CAD build for the part. Positions are in the model's coordinates, mm. Face numbers are marked on the shaded views. A direction names the side the tool comes from. Round coordinates to 2 decimals unless told otherwise and drop trailing zeros. Write each loop counter-clockwise with the first axis right and the second up, starting at its lowest first coordinate (ties: lowest second). Pieces come first, ordered by that corner, then holes. Notation, with made-up numbers: (41, 38.5) - (69, 38.5) arc R12 ccw to (69, 55.5) - close; hole circle Ø4 at (-40, 25). An arc over 180 degrees is marked (long way). Answer in a Markdown table with one row per item.
```python
from build123d import *

# Parameters (mm, degrees)
MOTOR_MOUNT_SOLID_DEPTH              = 7.5
ENCODER_DISTANCE_SKETCH_W            = 50
ENCODER_DISTANCE_SKETCH_H            = 55
ENCODER_DISTANCE_SOLID_DEPTH         = 5
ENCODER_MOUNT_SKETCH_R               = 1.9
ENCODER_MOUNT_SKETCH_W               = 7
ENCODER_MOUNT_SKETCH_H               = 9
ENCODER_MOUNT_SOLID_DEPTH            = 5
MOTOR_CLAMP_MOUNTING_HOLES_SKETCH_R  = 1.9
MOTOR_CLAMP_MOUNTING_HOLES_CUT_DEPTH = 16
GUSSET_PLATE_SKETCH_W                = 50
GUSSET_PLATE_SKETCH_H                = 5
GUSSET_PLATE_SOLID_DEPTH             = 16.5
GUSSET_SOLID_DEPTH                   = 1.5
MOUNTING_PLATE_SKETCH_W              = 50
MOUNTING_PLATE_SKETCH_H              = 92
MOUNTING_PLATE_SKETCH_R              = 2.65
MOUNTING_PLATE_SOLID_DEPTH           = 5
MOUNTING_HOLES_CUT_DEPTH             = 100.036609393
MOUNTING_HOLES_CUT_DEPTH_BACK        = 100.036609393
MOUNTING_HOLE_SKETCH_R               = 2.65
MOUNTING_PLATE_TRIM_SKETCH_W         = 50
MOUNTING_PLATE_TRIM_SKETCH_H         = 15.5
MOUNTING_PLATE_TRIM_SKETCH_H_2       = 40
MOUNTING_PLATE_TRIM_SKETCH_W_2       = 23.5
MOUNTING_PLATE_TRIM_SKETCH_H_3       = 16.5
MOUNTING_PLATE_TRIM_CUT_DEPTH        = 2


with BuildPart() as part:
    # Mouting Mount Sketch → Motor Mount Solid (new, symmetric)
    with BuildSketch(Plane.XY):
        with BuildLine():
            Line((-25, -55), (25, -55))
            Line((25, -55), (25, 0))
            Line((25, 0), (10, 0))
            ThreePointArc((10, 0), (0, -10), (-10, 0))
            Line((-10, 0), (-25, 0))
            Line((-25, 0), (-25, -55))
        make_face()
    extrude(amount=MOTOR_MOUNT_SOLID_DEPTH, both=True)

    # Encoder Distance Sketch → Encoder Distance Solid (add)
    with BuildSketch(Plane.XZ.offset(55)):
        with Locations((0, 20)):
            Rectangle(ENCODER_DISTANCE_SKETCH_W, ENCODER_DISTANCE_SKETCH_H)
    extrude(amount=ENCODER_DISTANCE_SOLID_DEPTH)

    # Encoder Mount Sketch → Encoder Mount Solid (add)
    with BuildSketch(Plane.XY.offset(47.5)):
        Polygon((-25, -60), (-25, -55), (-11.5, 11.5), (11.5, 11.5), (25, -55), (25, -60), align=None)
        with Locations((-8, 8)):
            Circle(ENCODER_MOUNT_SKETCH_R, mode=Mode.SUBTRACT)
        with Locations((8, 8)):
            Circle(ENCODER_MOUNT_SKETCH_R, mode=Mode.SUBTRACT)
        with Locations((-8, -8)):
            Circle(ENCODER_MOUNT_SKETCH_R, mode=Mode.SUBTRACT)
        with Locations((8, -8)):
            Circle(ENCODER_MOUNT_SKETCH_R, mode=Mode.SUBTRACT)
        with Locations((-8, 0)):
            Rectangle(ENCODER_MOUNT_SKETCH_W, ENCODER_MOUNT_SKETCH_H, mode=Mode.SUBTRACT)
        with Locations((8, 0)):
            Rectangle(ENCODER_MOUNT_SKETCH_W, ENCODER_MOUNT_SKETCH_H, mode=Mode.SUBTRACT)
    extrude(amount=ENCODER_MOUNT_SOLID_DEPTH)

    # Motor Clamp Mounting Holes Sketch → Motor Clamp Mounting Holes Cut (cut)
    with BuildSketch(Plane(origin=(0, 0, 0), x_dir=(1, 0, 0), z_dir=(0, 1, 0))):
        with Locations(Location((-15, 0, 0), (0, 0, 180))):
            Circle(MOTOR_CLAMP_MOUNTING_HOLES_SKETCH_R)
        with Locations(Location((15, 0, 0), (0, 0, 180))):
            Circle(MOTOR_CLAMP_MOUNTING_HOLES_SKETCH_R)
    extrude(amount=-MOTOR_CLAMP_MOUNTING_HOLES_CUT_DEPTH, mode=Mode.SUBTRACT)

    # Gusset Plate Sketch → Gusset Plate Solid (add)
    with BuildSketch(Plane.XY.offset(52.5)):
        with Locations((0, -57.5)):
            Rectangle(GUSSET_PLATE_SKETCH_W, GUSSET_PLATE_SKETCH_H)
    extrude(amount=GUSSET_PLATE_SOLID_DEPTH)

    # Gusset Sketch → Gusset Solid (add, symmetric)
    with BuildSketch(Plane(origin=(0, 0, 0), x_dir=(0, 0, -1), z_dir=(1, 0, 0))):
        Polygon((-52.5, 11.5), (-69, -55), (-52.5, -55), align=None)
    extrude(amount=GUSSET_SOLID_DEPTH, both=True)

    # Mounting Plate Sketch → Mounting Plate Solid (add)
    with BuildSketch(Plane(origin=(0, -55, 0), x_dir=(1, 0, 0), z_dir=(0, 1, 0))):
        with Locations((0, -23)):
            Rectangle(MOUNTING_PLATE_SKETCH_W, MOUNTING_PLATE_SKETCH_H)
        with Locations((-19, -63)):
            Circle(MOUNTING_PLATE_SKETCH_R, mode=Mode.SUBTRACT)
        with Locations((19, -63)):
            Circle(MOUNTING_PLATE_SKETCH_R, mode=Mode.SUBTRACT)
        with Locations(Location((-19, 17, 0), (0, 0, 270))):
            Circle(MOUNTING_PLATE_SKETCH_R, mode=Mode.SUBTRACT)
        with Locations(Location((19, 17, 0), (0, 0, 270))):
            Circle(MOUNTING_PLATE_SKETCH_R, mode=Mode.SUBTRACT)
    extrude(amount=-MOUNTING_PLATE_SOLID_DEPTH)

    # Mounting Hole Sketch → Mounting Holes Cut (cut, two sides: drawn at the far end of the back side and taken through both)
    with BuildSketch(Plane(origin=(0, -55, 0), x_dir=(1, 0, 0), z_dir=(0, 1, 0)).offset(-MOUNTING_HOLES_CUT_DEPTH_BACK)):
        with Locations(Location((-19, 17, 0), (0, 0, 270))):
            Circle(MOUNTING_HOLE_SKETCH_R)
        with Locations(Location((19, 17, 0), (0, 0, 270))):
            Circle(MOUNTING_HOLE_SKETCH_R)
        with Locations(Location((19, -63, 0), (0, 0, 90))):
            Circle(MOUNTING_HOLE_SKETCH_R)
        with Locations(Location((-19, -63, 0), (0, 0, 90))):
            Circle(MOUNTING_HOLE_SKETCH_R)
    extrude(amount=MOUNTING_HOLES_CUT_DEPTH + MOUNTING_HOLES_CUT_DEPTH_BACK, mode=Mode.SUBTRACT)

    # Mounting Plate Trim Sketch → Mounting Plate Trim Cut (cut)
    with BuildSketch(Plane(origin=(0, -55, 0), x_dir=(1, 0, 0), z_dir=(0, 1, 0))):
        with Locations((0, 15.25)):
            Rectangle(MOUNTING_PLATE_TRIM_SKETCH_W, MOUNTING_PLATE_TRIM_SKETCH_H)
        with Locations((0, -27.5)):
            Rectangle(MOUNTING_PLATE_TRIM_SKETCH_W, MOUNTING_PLATE_TRIM_SKETCH_H_2)
        with Locations((13.25, -60.75)):
            Rectangle(MOUNTING_PLATE_TRIM_SKETCH_W_2, MOUNTING_PLATE_TRIM_SKETCH_H_3)
        with Locations((-13.25, -60.75)):
            Rectangle(MOUNTING_PLATE_TRIM_SKETCH_W_2, MOUNTING_PLATE_TRIM_SKETCH_H_3)
    extrude(amount=-MOUNTING_PLATE_TRIM_CUT_DEPTH, mode=Mode.SUBTRACT)


solid = part.part
```
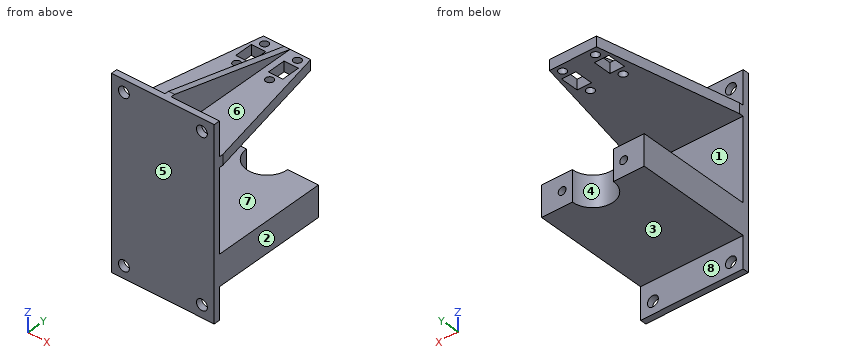
Q1. Drill centre lines: line 1 (Y direction, x = -8, z = 50); line 2 (Z direction, x = 12.5, y = -55); line 3 (X direction, y = -59.2, z = -17). Where is each one in solid material? Low to high.
Computed:
| item | result |
|---|---|
| line 1 | y = -60 to -9.9, -6.1 to -4.5, 4.5 to 6.1, 9.9 to 11.5 |
| line 2 | z = -7.5 to 7.5, 47.5 to 52.5 |
| line 3 | x = -25 to -21.65, -16.35 to 16.35, 21.65 to 25 |
Q2. Saw through at A-A on z = -17. List the corners of the cut face in (x, y).
Computed:
| item | result |
|---|---|
| outline | (-25, -60) - (-21.65, -60) - (-21.65, -57) - (-25, -57) - close; (-16.35, -60) - (16.35, -60) - (16.35, -57) - (-16.35, -57) - close; (21.65, -60) - (25, -60) - (25, -57) - (21.65, -57) - close |
Q3. Saw through at D-D on x = 0. List the corners of the cut face in (y, z).
Computed:
| item | result |
|---|---|
| outline | (-60, -23) - (-57, -23) - (-57, -7.5) - (-10, -7.5) - (-10, 7.5) - (-57, 7.5) - (-57, 47.5) - (11.5, 47.5) - (11.5, 52.5) - (-55, 69) - (-60, 69) - close |
Q4. Flat gauge pins, fed straight in: pin 1 (6 mm diameter, centred on x = -9, y = -23, fed in from -Z); pin 2 (16.5 mm diameter, centred on x = -14, z = -3, fed in from +Y); pin 3 (8 mm diameter, centred on y = -32.5, z = 58.5, fed in from -X). Where does each tip first touch, or does it go through?
Computed:
| item | result |
|---|---|
| pin 1 | stops at z = -7.5 |
| pin 2 | stops at y = 0 |
| pin 3 | stops at x = -1.5 |
Q5. Pull direction Z, two halves, no side cores. Call the marked faces 1, 2 and 3: released by +Z, released by -Z, zero draft, split by the parting line, or undercut.
Computed:
| item | result |
|---|---|
| face 1 | undercut |
| face 2 | zero draft |
| face 3 | released by -Z |
Q6. Saw through at C-C on y = -50. List the corners of the cut face in (x, z).
Computed:
| item | result |
|---|---|
| outline | (-25, -7.5) - (25, -7.5) - (25, 7.5) - (-25, 7.5) - close; (-23.98, 47.5) - (23.98, 47.5) - (23.98, 52.5) - (1.5, 52.5) - (1.5, 67.76) - (-1.5, 67.76) - (-1.5, 52.5) - (-23.98, 52.5) - close |
Q7. Saw through at B-B on x = -8. List the corners of the cut face in (y, z).
Computed:
| item | result |
|---|---|
| outline | (-60, -23) - (-57, -23) - (-57, -7.5) - (-6, -7.5) - (-6, 7.5) - (-57, 7.5) - (-57, 47.5) - (-9.9, 47.5) - (-9.9, 52.5) - (-57, 52.5) - (-57, 69) - (-60, 69) - close; (-6.1, 47.5) - (-4.5, 47.5) - (-4.5, 52.5) - (-6.1, 52.5) - close; (4.5, 47.5) - (6.1, 47.5) - (6.1, 52.5) - (4.5, 52.5) - close; (9.9, 47.5) - (11.5, 47.5) - (11.5, 52.5) - (9.9, 52.5) - close |
Q8. 3-axis set-ups, long thin cutter, end or side, ignore diameter. For the marked faces 4, 5, 6, 7 and 8: which of +Z, -Z, +X, -X, +Y, -Y reach the whole face in a straight line?
Computed:
| item | result |
|---|---|
| face 4 | -Z, +Y |
| face 5 | +Z, -Z, +X, -X, -Y |
| face 6 | +Z, +X, +Y |
| face 7 | +X, -X, +Y |
| face 8 | -Z, +X, -X, +Y |
